Could you check a few things on this drawing? It's one solid part, dimensions in mm from its lowest x, y, z. A direction names the side the tool comes from. Round coordinates to 2 decimals unless told otherwise and drop trailing zeros. Loops run counter-clockwise (first coordinate to the right, second up) from the corner with the lowest first, then second, coordinate; pieces in that order, holes last. Notation, with made-up numbers: (-26.5, 58) -> (-20.5, 58) arc R33 ccw to (-20.5, 97) -> close; hole circle Ø4 at (-12.5, 65.5). An arc over 180 degrees is marked (long way). Put each result on its own line as item: value. Start each with the question number.
1. I need wall thicknesses on line 1 (X direction, y = 4.5, z = 25.5). Which ranges of the line are inside material? Lowest first, please. Write a range as [from, to].
2. Imagine slicing it at C-C, the plane y = 11. Please give me the cut outline in (x, z), and give its area (3 significant figures).
3. If we mould it in two halves opening along X, with no side actions, what happens to the marked faces 1, 2 and 3? For each: pulls with the +X half, pulls with the -X half, needs draft (parallel to the pull), parting line crosses it, or undercut.
4. Imagine slicing it at B-B, the plane z = 49. Please give me the cut outline in (x, y).
5. Which directions (+Z, -Z, +X, -X, +Y, -Y) give clear straight access to the entire face, cutting with the end or side of a thin tool? Please do the marked faces 4 and 5.
6. Imagine slicing it at A-A, the plane x = 38. Please give me the cut outline in (y, z).
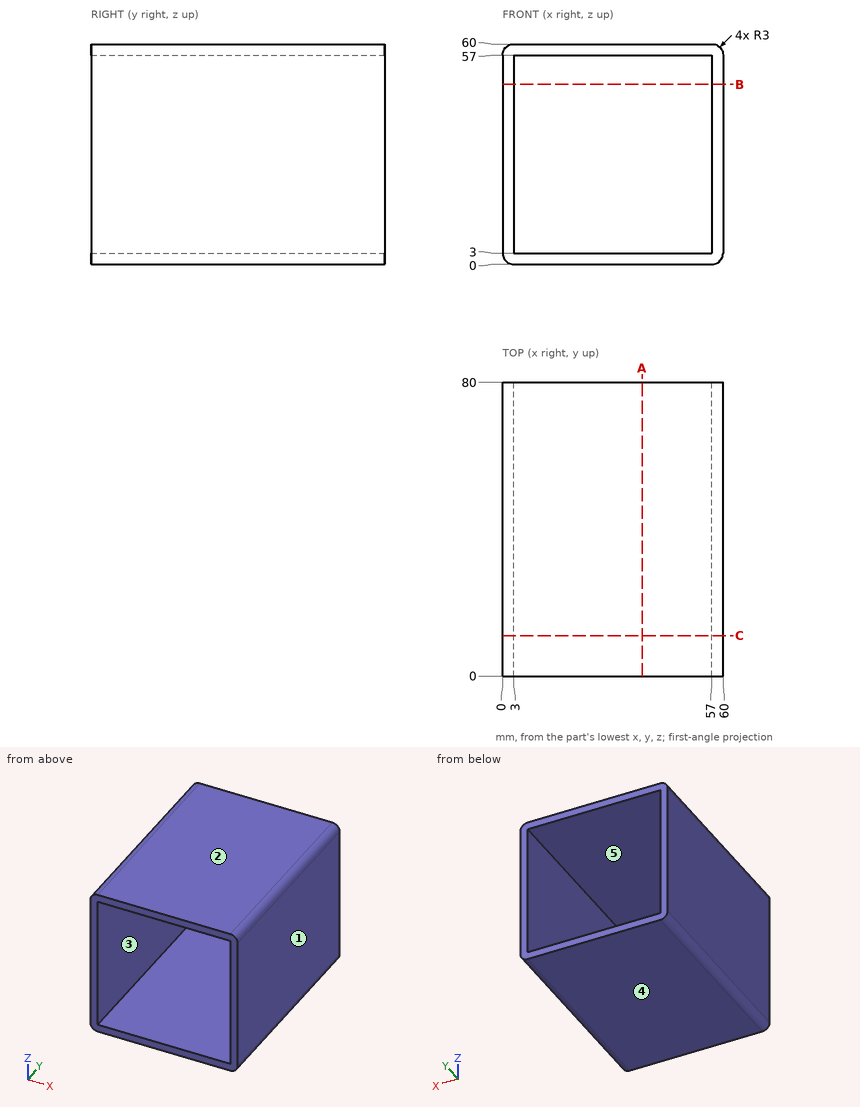
Entries:
1. line 1: [0, 3], [57, 60]
2. outline: (0, 3) arc R3 ccw to (3, 0) -> (57, 0) arc R3 ccw to (60, 3) -> (60, 57) arc R3 ccw to (57, 60) -> (3, 60) arc R3 ccw to (0, 57) -> close; hole (3, 3) -> (57, 3) -> (57, 57) -> (3, 57) -> close
2. area: 676 mm^2
3. face 1: pulls with the +X half
3. face 2: needs draft
3. face 3: undercut
4. outline: (0, 0) -> (3, 0) -> (3, 80) -> (0, 80) -> close; (57, 0) -> (60, 0) -> (60, 80) -> (57, 80) -> close
5. face 4: -Z, +X, -X, +Y, -Y
5. face 5: +Y, -Y
6. outline: (0, 0) -> (80, 0) -> (80, 3) -> (0, 3) -> close; (0, 57) -> (80, 57) -> (80, 60) -> (0, 60) -> close
